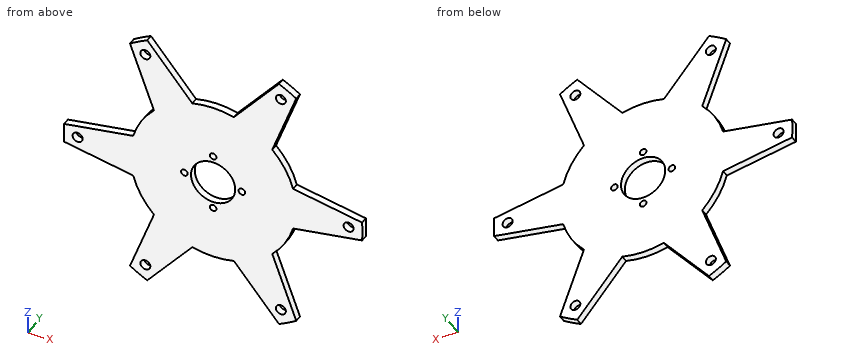
```python
from build123d import *

# Parameters (mm, degrees)
SKETCH2_R           = 10
SKETCH2_R_2         = 1.5
SKETCH2_R_3         = 2.25
BOSS_EXTRUDE1_DEPTH = 3.175


with BuildPart() as part:
    # Sketch2 → Boss-Extrude1 (new body)
    with BuildSketch(Plane(origin=(0, 0, 0), x_dir=(1, 0, 0), z_dir=(0, 1, 0))):
        with BuildLine():
            Line((-36.142080737, 10), (-67.350020101, 4.497198278))
            ThreePointArc((-67.350020101, 4.497198278), (-67.5, 0), (-67.350020101, -4.497198278))
            Line((-67.350020101, -4.497198278), (-36.142080737, -10))
            ThreePointArc((-36.142080737, -10), (-32.475952642, -18.75), (-26.731294406, -26.299960064))
            Line((-26.731294406, -26.299960064), (-37.569698005, -56.078229214))
            ThreePointArc((-37.569698005, -56.078229214), (-33.75, -58.456714755), (-29.780322096, -60.575427492))
            Line((-29.780322096, -60.575427492), (-9.410786331, -36.299960064))
            ThreePointArc((-9.410786331, -36.299960064), (0, -37.5), (9.410786331, -36.299960064))
            Line((9.410786331, -36.299960064), (29.780322096, -60.575427492))
            ThreePointArc((29.780322096, -60.575427492), (33.75, -58.456714755), (37.569698005, -56.078229214))
            Line((37.569698005, -56.078229214), (26.731294406, -26.299960064))
            ThreePointArc((26.731294406, -26.299960064), (32.475952642, -18.75), (36.142080737, -10))
            Line((36.142080737, -10), (67.350020101, -4.497198278))
            ThreePointArc((67.350020101, -4.497198278), (67.5, 0), (67.350020101, 4.497198278))
            Line((67.350020101, 4.497198278), (36.142080737, 10))
            ThreePointArc((36.142080737, 10), (32.475952642, 18.75), (26.731294406, 26.299960064))
            Line((26.731294406, 26.299960064), (37.569698005, 56.078229214))
            ThreePointArc((37.569698005, 56.078229214), (33.75, 58.456714755), (29.780322096, 60.575427492))
            Line((29.780322096, 60.575427492), (9.410786331, 36.299960064))
            ThreePointArc((9.410786331, 36.299960064), (0, 37.5), (-9.410786331, 36.299960064))
            Line((-9.410786331, 36.299960064), (-29.780322096, 60.575427492))
            ThreePointArc((-29.780322096, 60.575427492), (-33.75, 58.456714755), (-37.569698005, 56.078229214))
            Line((-37.569698005, 56.078229214), (-26.731294406, 26.299960064))
            ThreePointArc((-26.731294406, 26.299960064), (-32.475952642, 18.75), (-36.142080737, 10))
        make_face()
        with Locations(Location((0, 0, 0), (0, 0, 270))):
            Circle(SKETCH2_R, mode=Mode.SUBTRACT)
        with Locations(Location((0, 13, 0), (0, 0, 270))):
            Circle(SKETCH2_R_2, mode=Mode.SUBTRACT)
        with Locations(Location((13, 0, 0), (0, 0, 270))):
            Circle(SKETCH2_R_2, mode=Mode.SUBTRACT)
        with Locations(Location((0, -13, 0), (0, 0, 270))):
            Circle(SKETCH2_R_2, mode=Mode.SUBTRACT)
        with Locations(Location((-13, 0, 0), (0, 0, 270))):
            Circle(SKETCH2_R_2, mode=Mode.SUBTRACT)
        with Locations(Location((-61.25, 0, 0), (0, 0, 270))):
            Circle(SKETCH2_R_3, mode=Mode.SUBTRACT)
        with Locations(Location((-30.625, 53.044055982, 0), (0, 0, 270))):
            Circle(SKETCH2_R_3, mode=Mode.SUBTRACT)
        with Locations(Location((30.625, 53.044055982, 0), (0, 0, 270))):
            Circle(SKETCH2_R_3, mode=Mode.SUBTRACT)
        with Locations(Location((61.25, 0, 0), (0, 0, 270))):
            Circle(SKETCH2_R_3, mode=Mode.SUBTRACT)
        with Locations(Location((30.625, -53.044055982, 0), (0, 0, 270))):
            Circle(SKETCH2_R_3, mode=Mode.SUBTRACT)
        with Locations(Location((-30.625, -53.044055982, 0), (0, 0, 270))):
            Circle(SKETCH2_R_3, mode=Mode.SUBTRACT)
    extrude(amount=BOSS_EXTRUDE1_DEPTH)


solid = part.part
```
Could you check a few things on this model? Use its own coordinates, in mm. Coordinates: 2 decimals unless noted, no trailing zeros. Loops run counter-clockwise (first coordinate to the right, second up) from the corner with the lowest first, then second, coordinate; pieces in that order, holes last.
1) Will these pins go through, and if not, where does the flat tip stop? pin 1 Ø6 at (x, z) = (30.62, 53.04) entering from -Y; pin 2 Ø1 at (y, z) = (2, 4) entering from +X.
Reported:
pin 1: stops at y = 0
pin 2: stops at x = 67.41
2) Please list where these lines run through material, in increasing order: line 1 along X through (y, z) = (2.4, 0); line 2 along X through (y, z) = (2.1, -51); line 3 along X through (y, z) = (0.3, 45).
Reported:
line 1: x = -67.5 to -63.5, -59 to -14.5, -11.5 to -10, 10 to 11.5, 14.5 to 59, 63.5 to 67.5
line 2: x = -35.72 to -31.57, -29.68 to -21.75, 21.75 to 29.68, 31.57 to 35.72
line 3: x = -33.54 to -16.71, 16.71 to 33.54
3) Imagine slicing it at B-B (z = -47). List the corners of the cut face in (x, y) for me (1 decimal).
Reported:
outline: (-34.3, 0) - (-18.4, 0) - (-18.4, 3.2) - (-34.3, 3.2) - close; (18.4, 0) - (34.3, 0) - (34.3, 3.2) - (18.4, 3.2) - close
4) Imagine slicing it at D-D (y = 0.7). State how many separate pieces and enclosed holes the cut face has, and give its area (3 significant figures).
Reported:
separate pieces: 1
enclosed holes: 11
area: 6,590 mm2
5) Imagine slicing it at C-C (x = -61.25). List the corners of the cut face in (y, z) for me (3 decimals), and give its area (3 significant figures).
Reported:
outline: (0, -5.573) - (3.175, -5.573) - (3.175, -2.25) - (0, -2.25) - close; (0, 2.25) - (3.175, 2.25) - (3.175, 5.573) - (0, 5.573) - close
area: 21.1 mm2
6) Imagine slicing it at A-A (x = 0). List the corners of the cut face in (y, z) for me (3 decimals), and give its area (3 significant figures).
Reported:
outline: (0, -37.5) - (3.175, -37.5) - (3.175, -14.5) - (0, -14.5) - close; (0, -11.5) - (3.175, -11.5) - (3.175, -10) - (0, -10) - close; (0, 10) - (3.175, 10) - (3.175, 11.5) - (0, 11.5) - close; (0, 14.5) - (3.175, 14.5) - (3.175, 37.5) - (0, 37.5) - close
area: 156 mm2
